Design review of the part shown in the three views and the two pictorial views. Dimensions are in mm from the part's minimum x, y and z. A direction names the side the tool comes from. Round coordinates to 2 decimals unless told otherwise and drop trailing zeros. Loops run counter-clockwise (first coordinate to the right, second up) from the corner with the lowest first, then second, coordinate; pieces in that order, holes last. Notation, with made-up numbers: M 58,4 L 95,4 A10 ccw 95,20 Z; hole C -16,63.5 d3. An arc over 180 degrees is marked long. Return JSON: item names as keys, results as strings. Group by question number.
Q1. Consider section A-A (x = 1.85). State the section outline as (y, z) points.
Q2. Clearance check with flat-ended pins moving along their axes: pin 1 Ø1 at (y, z) = (8, 4) entering from +X; pin 2 Ø1.6 at (y, z) = (17, 5.5) entering from -X; pin 3 Ø3 at (x, z) = (25.35, 4.25) entering from +Y; pin 4 Ø4 at (y, z) = (16.5, 7) entering from +X. State where each tip first meets the part, or that it passes through.
Q3. For the marked faces 1, 2, 3, 4 and 5, list the 3-axis set-ups (+Z, -Z, +X, -X, +Y, -Y) from which the entire face can be reached by the end or side of a thin tool; tool diameter is ignored.
Q4. Consider section C-C (y = 8.5). State the section outline as (x, z) points, and give its area (3 significant figures).
Q5. Consider section B-B (z = 8). State the section outline as (x, y) points.
Q6. To check wall thickness, follow line 1 along X through (y, z) = (15.35, 4.25); line 2 along Z through (x, y) = (25.35, 15.55); line 3 along X through (y, z) = (15.8, 4.25). State the ranges of each line that lie inside material, in increasing order.
Q7. Consider section D-D (x = 5.5). State the section outline as (y, z) points, and give its area (3 significant figures).
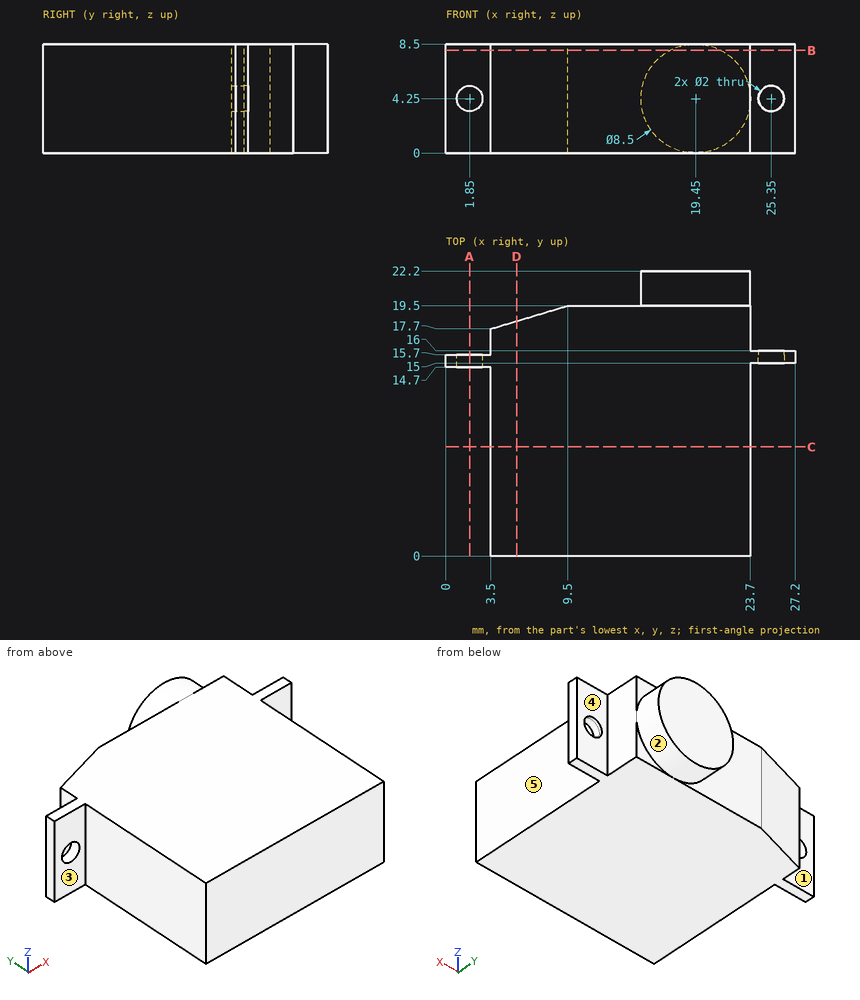
Values:
{
 "1": {"outline": "M 14.7,0 L 15.7,0 L 15.7,3.25 L 14.7,3.25 Z; M 14.7,5.25 L 15.7,5.25 L 15.7,8.5 L 14.7,8.5 Z"},
 "2": {"pin 1": "stops at x = 23.7", "pin 2": "stops at x = 3.5", "pin 3": "stops at y = 16", "pin 4": "stops at x = 27.2"},
 "3": {"face 1": "+Z, -Z, -X, +Y", "face 2": "+Y", "face 3": "+Z, -Z, -X, -Y", "face 4": "+Z, -Z, +X, +Y", "face 5": "+Z, -Z, +X, -Y"},
 "4": {"outline": "M 3.5,0 L 23.7,0 L 23.7,8.5 L 3.5,8.5 Z", "area": "172 mm2"},
 "5": {"outline": "M 0,14.7 L 3.5,14.7 L 3.5,0 L 23.7,0 L 23.7,15 L 27.2,15 L 27.2,16 L 23.7,16 L 23.7,19.5 L 21.45,19.5 L 21.45,22.2 L 17.45,22.2 L 17.45,19.5 L 9.5,19.5 L 3.5,17.7 L 3.5,15.7 L 0,15.7 Z"},
 "6": {"line 1": "x = 0 to 0.85, 2.85 to 24.35, 26.35 to 27.2", "line 2": "z = 0 to 3.25, 5.25 to 8.5", "line 3": "x = 3.5 to 24.35, 26.35 to 27.2"},
 "7": {"outline": "M 0,0 L 18.3,0 L 18.3,8.5 L 0,8.5 Z", "area": "156 mm2"}
}
